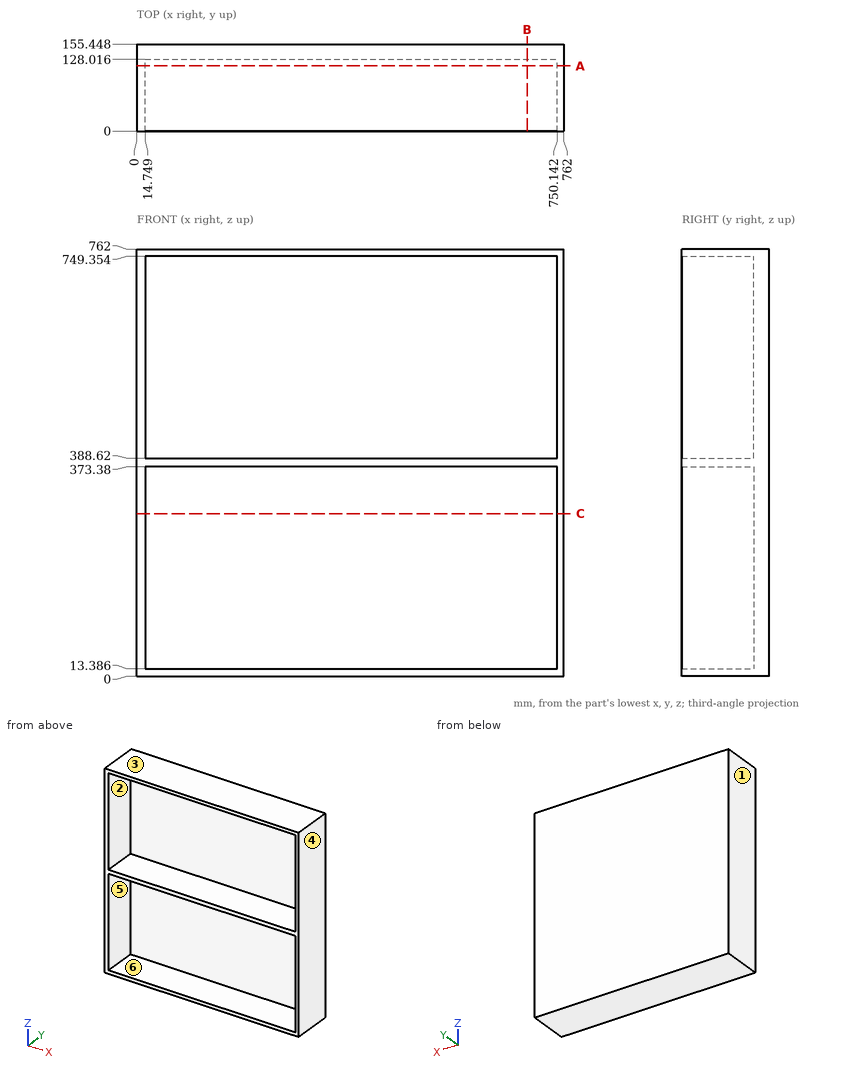
Design review of the part shown in the three views and the two pictorial views. Dimensions are in mm from the part's minimum x, y and z. A direction names the side the tool comes from. Round coordinates to 2 decimals unless told otherwise and drop trailing zeros. Loops run counter-clockwise (first coordinate to the right, second up) from the corner with the lowest first, then second, coordinate; pieces in that order, holes last. Notation, with made-up numbers: (-26, 48) - (20, 48) arc R26 cw to (20, 86) - close; hole circle Ø6 at (70.5, 6.25). An arc over 180 degrees is marked (long way). Use one line per item in the form item = value.
1) We need section B-B on x = 696.5. Write out the cut boundary in (y, z) (1 decimal).
Solutions:
outline = (0, 0) - (155.4, 0) - (155.4, 762) - (0, 762) - (0, 749.4) - (128, 749.4) - (128, 388.6) - (0, 388.6) - (0, 373.4) - (128, 373.4) - (128, 13.4) - (0, 13.4) - close
2) Clearance check with flat-ended pins moving along their axes: P1, Ø3, axis at y = 80, z = 493.5, coming from the -X side; P2, Ø6, axis at x = 521, z = 417.5, coming from the -Y side. State where each tip first meets the part, or that it passes through.
Solutions:
P1 = 0
P2 = 128.02
3) Tool access review of the marked faces 1 and 2: name each direction out of +Z, -Z, +X, -X, +Y, -Y from which nothing blocks a thin tool from reaching the whole face with its end or side.
Solutions:
face_1 = +Z, -Z, -X, +Y, -Y
face_2 = -Y
4) Mouldability with a two-part tool opening along Z and no side actions: class the marked faces 3, 4, 5 and 6 as pulls with the +Z half, pulls with the -Z half, needs draft (parallel to the pull), parting line crosses it, or undercut.
Solutions:
face_3 = pulls with the +Z half
face_4 = needs draft
face_5 = undercut
face_6 = undercut
5) We need section C-C on z = 290. Write out the cut boundary in (x, y).
Solutions:
outline = (0, 0) - (14.75, 0) - (14.75, 128.02) - (750.14, 128.02) - (750.14, 0) - (762, 0) - (762, 155.45) - (0, 155.45) - close
6) Wall thickness on probe 1 along Z at (x, y) = (75.5, 33) (1 decimal); probe 2 along X at (y, z) = (16, 296); probe 3 along Y at (x, z) = (288.5, 158): over which ranges is each line inside the solid? List them lowest first.
Solutions:
probe_1 = 0 to 13.4, 373.4 to 388.6, 749.4 to 762
probe_2 = 0 to 14.75, 750.14 to 762
probe_3 = 128.02 to 155.45
7) We need section A-A on y = 116.5. State how many separate pieces and enclosed holes the cut face has, then the cut area to 3 significant figures.
Solutions:
separate_pieces = 1
enclosed_holes = 2
area = 50,600 mm2
